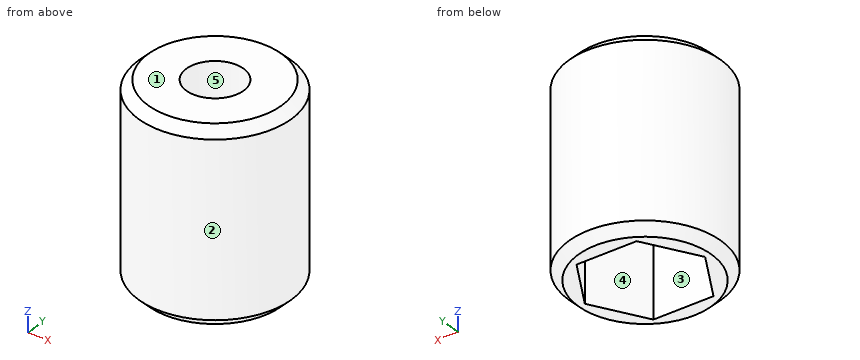
from build123d import *

# Parameters (mm, degrees)
ESQUISSE1_R             = 4
BASE_EXTRUSION_DEPTH    = 10
CHANFREIN1_SIZE         = 0.5
ESQUISSE2_R             = 1.5
ENL_V_MAT_EXTRU_1_DEPTH = 12.489125293
ENL_V_MAT_EXTRU_2_DEPTH = 6


with BuildPart() as part:
    # Esquisse1 → Base-Extrusion (new body)
    with BuildSketch(Plane.XY):
        Circle(ESQUISSE1_R)
    extrude(amount=BASE_EXTRUSION_DEPTH)

    # Chanfrein1
    chanfrein1_edges = [part.edges().sort_by_distance(p)[0] for p in [
        (-4, 0, 0),
        (-4, 0, 10),
    ]]
    chamfer(chanfrein1_edges, length=CHANFREIN1_SIZE)

    # Esquisse2 → Enlèv. mat.-Extru.1 (cut, through all)
    with BuildSketch(Plane.XY.offset(10)):
        Circle(ESQUISSE2_R)
    extrude(amount=-ENL_V_MAT_EXTRU_1_DEPTH, mode=Mode.SUBTRACT)

    # Esquisse3 → Enlèv. mat.-Extru.2 (cut)
    with BuildSketch(Plane(origin=(0, 0, 0), x_dir=(-1, 0, 0), z_dir=(0, 0, -1))):
        Polygon((1.58113883, 2.738612788), (-1.58113883, 2.738612788), (-3.16227766, 0), (-1.58113883, -2.738612788), (1.58113883, -2.738612788), (3.16227766, 0), align=None)
    extrude(amount=-ENL_V_MAT_EXTRU_2_DEPTH, mode=Mode.SUBTRACT)


solid = part.part
For this review, take the finished solid that the model builds, in its own axes (mm). Face numbers are marked on the shaded views. A direction names the side the tool comes from. Give positions to 0.01 mm unless a question says otherwise; leave off trailing zeros. Loops run counter-clockwise (first coordinate to the right, second up) from the corner with the lowest first, then second, coordinate; pieces in that order, holes last.
Item 1: For line 1 along Y through (x, z) = (0, 8.7); line 2 along X through (y, z) = (-0.5, 6.5); line 3 along X through (y, z) = (0.5, 2.25), list the stretches that pass through material, from the lowest coordinate up.
Item 2: Take a section at B-B, the plane z = 1. State the section outline as (x, y) points, and give its area (3 significant figures).
Item 3: Take a section at A-A, the plane x = 0. State the section outline as (y, z) points.
Item 4: Draft analysis for pull direction Y (two halves, no side actions). For the marked faces 1, 2 and 3, state which applies: +Y half, -Y half, draft (parallel to the pull), parting line (faces both ways), or undercut.
Item 5: Tool access review of the marked faces 4 and 5: name each direction out of +Z, -Z, +X, -X, +Y, -Y from which nothing blocks a thin tool from reaching the whole face with its end or side.
Item 6: Take a section at C-C, the plane z = 7.25. State the section outline as (x, y) points, and give its area (3 significant figures).
Calculated:
1. line 1: y = -4 to -1.5, 1.5 to 4
1. line 2: x = -3.97 to -1.41, 1.41 to 3.97
1. line 3: x = -3.97 to -2.87, 2.87 to 3.97
2. outline: circle Ø8 at (0, 0); hole (-3.16, 0) - (-1.58, -2.74) - (1.58, -2.74) - (3.16, 0) - (1.58, 2.74) - (-1.58, 2.74) - close
2. area: 24.3 mm2
3. outline: (-4, 0.5) - (-3.5, 0) - (-2.74, 0) - (-2.74, 6) - (-1.5, 6) - (-1.5, 10) - (-3.5, 10) - (-4, 9.5) - close; (1.5, 6) - (2.74, 6) - (2.74, 0) - (3.5, 0) - (4, 0.5) - (4, 9.5) - (3.5, 10) - (1.5, 10) - close
4. face 1: draft
4. face 2: parting line
4. face 3: undercut
5. face 4: -Z
5. face 5: +Z, -Z
6. outline: circle Ø8 at (0, 0); hole circle Ø3 at (0, 0)
6. area: 43.2 mm2
